```python
from build123d import *

# Parameters (mm, degrees)
ESBO_O1_R                = 1.15
RESSALTO_EXTRUS_O1_DEPTH = 20
FILETE1_R                = 2


with BuildPart() as part:
    # Esboço1 → Ressalto-extrusão1 (new body)
    with BuildSketch(Plane(origin=(0, 0, 0), x_dir=(1, 0, 0), z_dir=(0, 1, 0))):
        with BuildLine():
            Line((-8.5, 9), (-8.5, 6))
            Line((-8.5, 6), (-26, 6))
            Line((-26, 6), (-26, -6))
            Line((-26, -6), (-8.5, -6))
            Line((-8.5, -6), (-8.5, -9))
            ThreePointArc((-8.5, -9), (-4.25, -13.25), (0, -9))
            Line((0, -9), (0, 9))
            ThreePointArc((0, 9), (-4.25, 13.25), (-8.5, 9))
        make_face()
        with Locations(Location((-4.25, 9, 0), (0, 0, 270))):
            Circle(ESBO_O1_R, mode=Mode.SUBTRACT)
        with Locations(Location((-4.25, -9, 0), (0, 0, 270))):
            Circle(ESBO_O1_R, mode=Mode.SUBTRACT)
    extrude(amount=RESSALTO_EXTRUS_O1_DEPTH)

    # Filete1
    filete1_edges = [part.edges().sort_by_distance(p)[0] for p in [
        (-8.5, 10, 6),
        (-26, 10, 6),
        (-26, 10, -6),
        (-8.5, 10, -6),
    ]]
    fillet(filete1_edges, radius=FILETE1_R)


solid = part.part
```
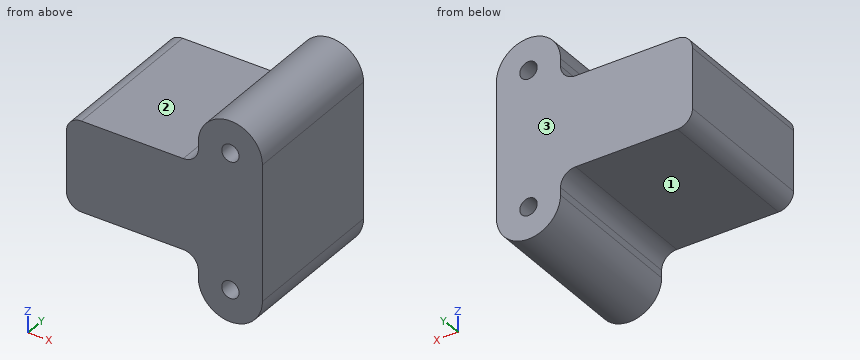
Verification items for the finished model (mm, model axes). Face numbers are marked on the shaded views. A direction names the side the tool comes from. Coordinates: 2 decimals unless noted, no trailing zeros. Loops run counter-clockwise (first coordinate to the right, second up) from the corner with the lowest first, then second, coordinate; pieces in that order, holes last. Notation, with made-up numbers: (25.5, 50) -> (46.5, 50) arc R18 ccw to (46.5, 76) -> close; hole circle Ø9 at (84, 64). An arc over 180 degrees is marked (long way). Answer in a Markdown table with one row per item.
1) Section check B-B (y = 2). Record the cut outline in (x, z).
The answers:
| item | result |
|---|---|
| outline | (-26, -4) arc R2 ccw to (-24, -6) -> (-10.5, -6) arc R2 cw to (-8.5, -8) -> (-8.5, -9) arc R4.25 ccw to (0, -9) -> (0, 9) arc R4.25 ccw to (-8.5, 9) -> (-8.5, 8) arc R2 cw to (-10.5, 6) -> (-24, 6) arc R2 ccw to (-26, 4) -> close; hole circle Ø2.3 at (-4.25, -9); hole circle Ø2.3 at (-4.25, 9) |
2) Section check A-A (x = -4.25). Record the cut outline in (y, z).
The answers:
| item | result |
|---|---|
| outline | (0, -13.25) -> (20, -13.25) -> (20, -10.15) -> (0, -10.15) -> close; (0, -7.85) -> (20, -7.85) -> (20, 7.85) -> (0, 7.85) -> close; (0, 10.15) -> (20, 10.15) -> (20, 13.25) -> (0, 13.25) -> close |
3) Depth check by flat-ended pin: P1, Ø1.5, axis at x = -13.5, y = 14, coming from the -Z side; P2, Ø1, axis at x = -15.5, y = 8, coming from the +Z side; P3, Ø0.8, axis at y = 8.5, z = 8.5, coming from the -X side. Enter the tip coordinate at first touch or a pass-through.
The answers:
| item | result |
|---|---|
| P1 | stops at z = -6 |
| P2 | stops at z = 6 |
| P3 | stops at x = -8.5 |
4) Scan lines: line 1 along X through (y, z) = (12.5, -9); line 2 along Z through (x, y) = (-4.5, 18.75); line 3 along Z through (x, y) = (-5, 13.75). Record each from-to range of solid material in increasing order. Write a range as from..to.
The answers:
| item | result |
|---|---|
| line 1 | x = -8.5..-5.4, -3.1..0 |
| line 2 | z = -13.24..-10.12, -7.88..7.88, 10.12..13.24 |
| line 3 | z = -13.18..-9.87, -8.13..8.13, 9.87..13.18 |
5) Section check C-C (z = 9.75). Record the cut outline in (x, y).
The answers:
| item | result |
|---|---|
| outline | (-8.43, 0) -> (-5.12, 0) -> (-5.12, 20) -> (-8.43, 20) -> close; (-3.38, 0) -> (-0.07, 0) -> (-0.07, 20) -> (-3.38, 20) -> close |
6) Access from +Z, -Z, +X, -X, +Y, -Y to the whole of each face (thin tool, end or side, straight path). Record for the marked faces 1, 2 and 3.
The answers:
| item | result |
|---|---|
| face 1 | -Z, -X, +Y, -Y |
| face 2 | +Z, -X, +Y, -Y |
| face 3 | +Z, -Z, +X, -X, +Y |
7) Section check D-D (x = -17.75). Record the cut outline in (y, z).
The answers:
| item | result |
|---|---|
| outline | (0, -6) -> (20, -6) -> (20, 6) -> (0, 6) -> close |
